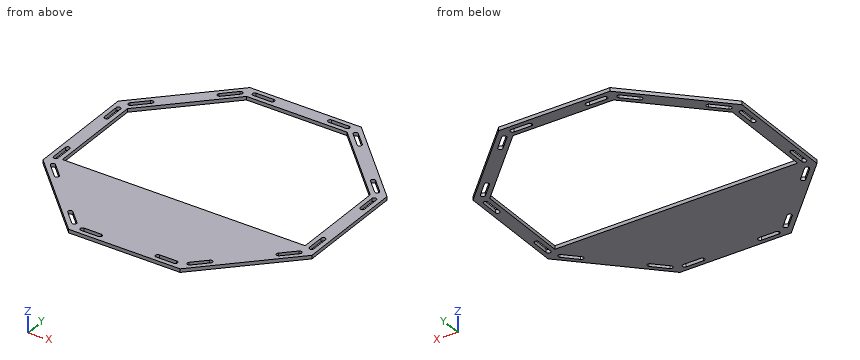
```python
from build123d import *

# Parameters (mm, degrees)
BOSS_EXTRUDE1_DEPTH     = 8
ENL_V_MAT_EXTRU_2_DEPTH = 10
ENL_V_MAT_EXTRU_3_DEPTH = 10


with BuildPart() as part:
    # Sketch1 → Boss-Extrude1 (new body)
    with BuildSketch(Plane.XY):
        Polygon((307.812229203, -127.5), (307.812229203, 127.5), (127.5, 307.812229203), (-127.5, 307.812229203), (-307.812229203, 127.5), (-307.812229203, -127.5), (-127.5, -307.812229203), (127.5, -307.812229203), align=None)
    extrude(amount=BOSS_EXTRUDE1_DEPTH)

    # Esquisse2 → Enlèv. mat.-Extru.2 (cut)
    with BuildSketch(Plane.XY.offset(8)):
        Polygon((-277.812229203, 115.073593129), (-277.812229203, -106.028471395), (277.812229203, -106.028471395), (277.812229203, 115.073593129), (115.073593129, 277.812229203), (-115.073593129, 277.812229203), align=None)
    extrude(amount=-ENL_V_MAT_EXTRU_2_DEPTH, mode=Mode.SUBTRACT)

    # Esquisse3 → Enlèv. mat.-Extru.3 (cut)
    with BuildSketch(Plane.XY.offset(8)):
        with BuildLine():
            Line((-285.725345882, 135.391380688), (-257.441074635, 163.675651935))
            ThreePointArc((-257.441074635, 163.675651935), (-250.370006823, 163.675651935), (-250.370006823, 156.604584124))
            Line((-250.370006823, 156.604584124), (-278.65427807, 128.320312876))
            ThreePointArc((-278.65427807, 128.320312876), (-285.725345882, 128.320312876), (-285.725345882, 135.391380688))
        make_face()
        with BuildLine():
            Line((-135.413116679, 285.703609891), (-163.697387927, 257.419338643))
            ThreePointArc((-163.697387927, 257.419338643), (-163.697387927, 250.348270831), (-156.626320115, 250.348270831))
            Line((-156.626320115, 250.348270831), (-128.342048868, 278.632542079))
            ThreePointArc((-128.342048868, 278.632542079), (-128.342048868, 285.703609891), (-135.413116679, 285.703609891))
        make_face()
        with BuildLine():
            Line((-106.270981056, 297.774677702), (-66.270981056, 297.774677702))
            ThreePointArc((-66.270981056, 297.774677702), (-61.270981056, 292.774677702), (-66.270981056, 287.774677702))
            Line((-66.270981056, 287.774677702), (-106.270981056, 287.774677702))
            ThreePointArc((-106.270981056, 287.774677702), (-111.270981056, 292.774677702), (-106.270981056, 297.774677702))
        make_face()
        with BuildLine():
            Line((106.302612073, 297.774677702), (66.302612073, 297.774677702))
            ThreePointArc((66.302612073, 297.774677702), (61.302612073, 292.774677702), (66.302612073, 287.774677702))
            Line((66.302612073, 287.774677702), (106.302612073, 287.774677702))
            ThreePointArc((106.302612073, 287.774677702), (111.302612073, 292.774677702), (106.302612073, 297.774677702))
        make_face()
        with BuildLine():
            Line((-297.796413694, 106.249245064), (-297.796413694, 66.249245064))
            ThreePointArc((-297.796413694, 66.249245064), (-292.796413694, 61.249245064), (-287.796413694, 66.249245064))
            Line((-287.796413694, 66.249245064), (-287.796413694, 106.249245064))
            ThreePointArc((-287.796413694, 106.249245064), (-292.796413694, 111.249245064), (-297.796413694, 106.249245064))
        make_face()
        with BuildLine():
            Line((-297.796413694, -106.324348065), (-297.796413694, -66.324348065))
            ThreePointArc((-297.796413694, -66.324348065), (-292.796413694, -61.324348065), (-287.796413694, -66.324348065))
            Line((-287.796413694, -66.324348065), (-287.796413694, -106.324348065))
            ThreePointArc((-287.796413694, -106.324348065), (-292.796413694, -111.324348065), (-297.796413694, -106.324348065))
        make_face()
        with BuildLine():
            Line((285.756976899, -135.466483688), (257.472705652, -163.750754936))
            ThreePointArc((257.472705652, -163.750754936), (250.40163784, -163.750754936), (250.40163784, -156.679687124))
            Line((250.40163784, -156.679687124), (278.685909088, -128.395415876))
            ThreePointArc((278.685909088, -128.395415876), (285.756976899, -128.395415876), (285.756976899, -135.466483688))
        make_face()
        with BuildLine():
            Line((135.444747697, -285.778712891), (163.729018944, -257.494441643))
            ThreePointArc((163.729018944, -257.494441643), (163.729018944, -250.423373832), (156.657951132, -250.423373832))
            Line((156.657951132, -250.423373832), (128.373679885, -278.707645079))
            ThreePointArc((128.373679885, -278.707645079), (128.373679885, -285.778712891), (135.444747697, -285.778712891))
        make_face()
        with BuildLine():
            Line((106.302612073, -297.849780703), (66.302612073, -297.849780703))
            ThreePointArc((66.302612073, -297.849780703), (61.302612073, -292.849780703), (66.302612073, -287.849780703))
            Line((66.302612073, -287.849780703), (106.302612073, -287.849780703))
            ThreePointArc((106.302612073, -287.849780703), (111.302612073, -292.849780703), (106.302612073, -297.849780703))
        make_face()
        with BuildLine():
            Line((-106.270981056, -297.849780703), (-66.270981056, -297.849780703))
            ThreePointArc((-66.270981056, -297.849780703), (-61.270981056, -292.849780703), (-66.270981056, -287.849780703))
            Line((-66.270981056, -287.849780703), (-106.270981056, -287.849780703))
            ThreePointArc((-106.270981056, -287.849780703), (-111.270981056, -292.849780703), (-106.270981056, -297.849780703))
        make_face()
        with BuildLine():
            Line((-135.413116679, -285.778712891), (-163.697387927, -257.494441643))
            ThreePointArc((-163.697387927, -257.494441643), (-163.697387927, -250.423373832), (-156.626320115, -250.423373832))
            Line((-156.626320115, -250.423373832), (-128.342048868, -278.707645079))
            ThreePointArc((-128.342048868, -278.707645079), (-128.342048868, -285.778712891), (-135.413116679, -285.778712891))
        make_face()
        with BuildLine():
            Line((-285.725345882, -135.466483688), (-257.441074635, -163.750754936))
            ThreePointArc((-257.441074635, -163.750754936), (-250.370006823, -163.750754936), (-250.370006823, -156.679687124))
            Line((-250.370006823, -156.679687124), (-278.65427807, -128.395415876))
            ThreePointArc((-278.65427807, -128.395415876), (-285.725345882, -128.395415876), (-285.725345882, -135.466483688))
        make_face()
        with BuildLine():
            Line((297.828044711, -106.324348065), (297.828044711, -66.324348065))
            ThreePointArc((297.828044711, -66.324348065), (292.828044711, -61.324348065), (287.828044711, -66.324348065))
            Line((287.828044711, -66.324348065), (287.828044711, -106.324348065))
            ThreePointArc((287.828044711, -106.324348065), (292.828044711, -111.324348065), (297.828044711, -106.324348065))
        make_face()
        with BuildLine():
            Line((297.828044711, 106.249245064), (297.828044711, 66.249245064))
            ThreePointArc((297.828044711, 66.249245064), (292.828044711, 61.249245064), (287.828044711, 66.249245064))
            Line((287.828044711, 66.249245064), (287.828044711, 106.249245064))
            ThreePointArc((287.828044711, 106.249245064), (292.828044711, 111.249245064), (297.828044711, 106.249245064))
        make_face()
        with BuildLine():
            Line((135.444747697, 285.703609891), (163.729018944, 257.419338643))
            ThreePointArc((163.729018944, 257.419338643), (163.729018944, 250.348270831), (156.657951132, 250.348270831))
            Line((156.657951132, 250.348270831), (128.373679885, 278.632542079))
            ThreePointArc((128.373679885, 278.632542079), (128.373679885, 285.703609891), (135.444747697, 285.703609891))
        make_face()
        with BuildLine():
            Line((285.756976899, 135.391380688), (257.472705652, 163.675651935))
            ThreePointArc((257.472705652, 163.675651935), (250.40163784, 163.675651935), (250.40163784, 156.604584124))
            Line((250.40163784, 156.604584124), (278.685909088, 128.320312876))
            ThreePointArc((278.685909088, 128.320312876), (285.756976899, 128.320312876), (285.756976899, 135.391380688))
        make_face()
    extrude(amount=-ENL_V_MAT_EXTRU_3_DEPTH, mode=Mode.SUBTRACT)


solid = part.part
```
Work out the finished part from the listing and answer in its coordinate system (mm). Give positions to 0.01 mm unless a question says otherwise; leave off trailing zeros. Write each loop counter-clockwise with the first axis right and the second up, starting at its lowest first coordinate (ties: lowest second). Pieces come first, ordered by that corner, then holes.
(1) Straight lines are drawn through the part: line 1 (X direction, y = 94, z = 7); line 2 (X direction, y = -256, z = 7); line 3 (Y direction, x = 26, z = 4.25). For each, find the intervals that lie inside material, in ascending order.
Final values:
line 1: x = -307.81 to -297.8, -287.8 to -277.81, 277.81 to 287.83, 297.83 to 307.81
line 2: x = -179.31 to -164.73, -151.05 to 151.08, 164.76 to 179.31
line 3: y = -307.81 to -106.03, 277.81 to 307.81
(2) The part is cut by section A-A on y = 78.5. Write down the section's boundary in (x, z).
Final values:
outline: (-307.81, 0) - (-297.8, 0) - (-297.8, 8) - (-307.81, 8) - close; (-287.8, 0) - (-277.81, 0) - (-277.81, 8) - (-287.8, 8) - close; (277.81, 0) - (287.83, 0) - (287.83, 8) - (277.81, 8) - close; (297.83, 0) - (307.81, 0) - (307.81, 8) - (297.83, 8) - close
(3) Flat-ended cylindrical pins translate along their axes: pin 1 Ø3 at (x, z) = (-193, 6) entering from +Y; pin 2 Ø2 at (y, z) = (215, 2) entering from -X; pin 3 Ø1.5 at (x, z) = (-242.5, 3) entering from -Y. Find the tip coordinate at first contact, or state that the pin passes through.
Final values:
pin 1: stops at y = 243.81
pin 2: stops at x = -221.31
pin 3: stops at y = -193.56
(4) The part is cut by section B-B on x = -50. Write down the section's boundary in (y, z), plus the area to 3 significant figures.
Final values:
outline: (-307.81, 0) - (-106.03, 0) - (-106.03, 8) - (-307.81, 8) - close; (277.81, 0) - (307.81, 0) - (307.81, 8) - (277.81, 8) - close
area: 1,850 mm2
(5) The part is cut by section D-D on y = -145. Write down the section's boundary in (x, z).
Final values:
outline: (-290.31, 0) - (-276.19, 0) - (-276.19, 8) - (-290.31, 8) - close; (-262.05, 0) - (262.08, 0) - (262.08, 8) - (-262.05, 8) - close; (276.22, 0) - (290.31, 0) - (290.31, 8) - (276.22, 8) - close
(6) The part is cut by section C-C on x = 74.5. Write down the section's boundary in (y, z).
Final values:
outline: (-307.81, 0) - (-297.85, 0) - (-297.85, 8) - (-307.81, 8) - close; (-287.85, 0) - (-106.03, 0) - (-106.03, 8) - (-287.85, 8) - close; (277.81, 0) - (287.77, 0) - (287.77, 8) - (277.81, 8) - close; (297.77, 0) - (307.81, 0) - (307.81, 8) - (297.77, 8) - close
